The model under review builds one solid part; all positions refer to its coordinate system, in mm. Coordinates: 2 decimals unless noted, no trailing zeros. Order: outer loops, then holes, each group sorted by start corner. A loop starts at its lowest first (then second) coordinate and runs counter-clockwise, first axis right, second up.
```python
from build123d import *

# Parameters (mm, degrees)
SKETCH_R        = 8
SKETCH_R_2      = 4
PAD_DEPTH       = 8
SKETCH001_R     = 2
HOLE_DEPTH      = 8
CHAMFER_SIZE    = 0.5
CHAMFER001_SIZE = 0.25


with BuildPart() as part:
    # Sketch → Pad (new body)
    with BuildSketch(Plane.XY):
        Circle(SKETCH_R)
        Circle(SKETCH_R_2, mode=Mode.SUBTRACT)
    extrude(amount=PAD_DEPTH)

    # Sketch001 → Hole (cut)
    with BuildSketch(Plane.XZ.offset(8)):
        with Locations((0, 4)):
            Circle(SKETCH001_R)
    extrude(amount=-HOLE_DEPTH, mode=Mode.SUBTRACT)

    # Chamfer
    chamfer_edges = [part.edges().sort_by_distance(p)[0] for p in [
        (-8, 0, 8),
        (-8, 0, 0),
        (-4, 0, 8),
        (-4, 0, 0),
    ]]
    chamfer(chamfer_edges, length=CHAMFER_SIZE)

    # Chamfer001
    chamfer001_edges = [part.edges().sort_by_distance(p)[0] for p in [
        (-1.414274, -7.873997, 2.585847),
        (-1.414274, -7.873997, 5.414153),
        (2, -7.745967, 4),
    ]]
    chamfer(chamfer001_edges, length=CHAMFER001_SIZE)


solid = part.part
```
(1) We need section B-B, the plane x = 0.25. Count the separate pieces of the cut face and the enclosed holes in it, and give its area (3 significant figures).
A:
separate pieces: 3
enclosed holes: 0
area: 47.1 mm2
(2) We need section A-A, the plane y = 0. Write out the cut boundary in (x, z), and give its area (3 significant figures).
A:
outline: (-8, 0.5) - (-7.5, 0) - (-4.5, 0) - (-4, 0.5) - (-4, 7.5) - (-4.5, 8) - (-7.5, 8) - (-8, 7.5) - close; (4, 0.5) - (4.5, 0) - (7.5, 0) - (8, 0.5) - (8, 7.5) - (7.5, 8) - (4.5, 8) - (4, 7.5) - close
area: 63.0 mm2
(3) For pin 1 Ø2 at (x, z) = (3.5, 6.5) entering from -Y; pin 2 Ø1 at (y, z) = (-5, 3.5) entering from -X; pin 3 Ø2.5 at (x, z) = (0, 4) entering from -Y; pin 4 Ø1 at (x, y) = (-4.5, -3.5) entering from -Z, all flat-tipped, find the tip position at first contact; note any pin that passes through.
A:
pin 1: stops at y = -7.6
pin 2: stops at x = -6.61
pin 3: stops at y = 3.8
pin 4: stops at z = 0
(4) Wall thickness on probe 1 along Y at (x, z) = (0, 4.5); probe 2 along Z at (x, y) = (0, -5.8); probe 3 along X at (y, z) = (3, 3.75): over which ranges is each line inside the solid? List them lowest first.
A:
probe 1: y = 4 to 8
probe 2: z = 0 to 2, 6 to 8
probe 3: x = -7.42 to -2.65, 2.65 to 7.42
(5) Draft analysis for pull direction X (two halves, no side actions). For faces 1 (the face through (0, -5, 8)), 2 (the face through (4.301, 6.746, 3.951)), 3 (the face through (-2, -6, 4)), state which applies: released by +X, released by -X, zero draft, split by the parting line, or undercut.
A:
face 1: zero draft
face 2: split by the parting line
face 3: undercut
